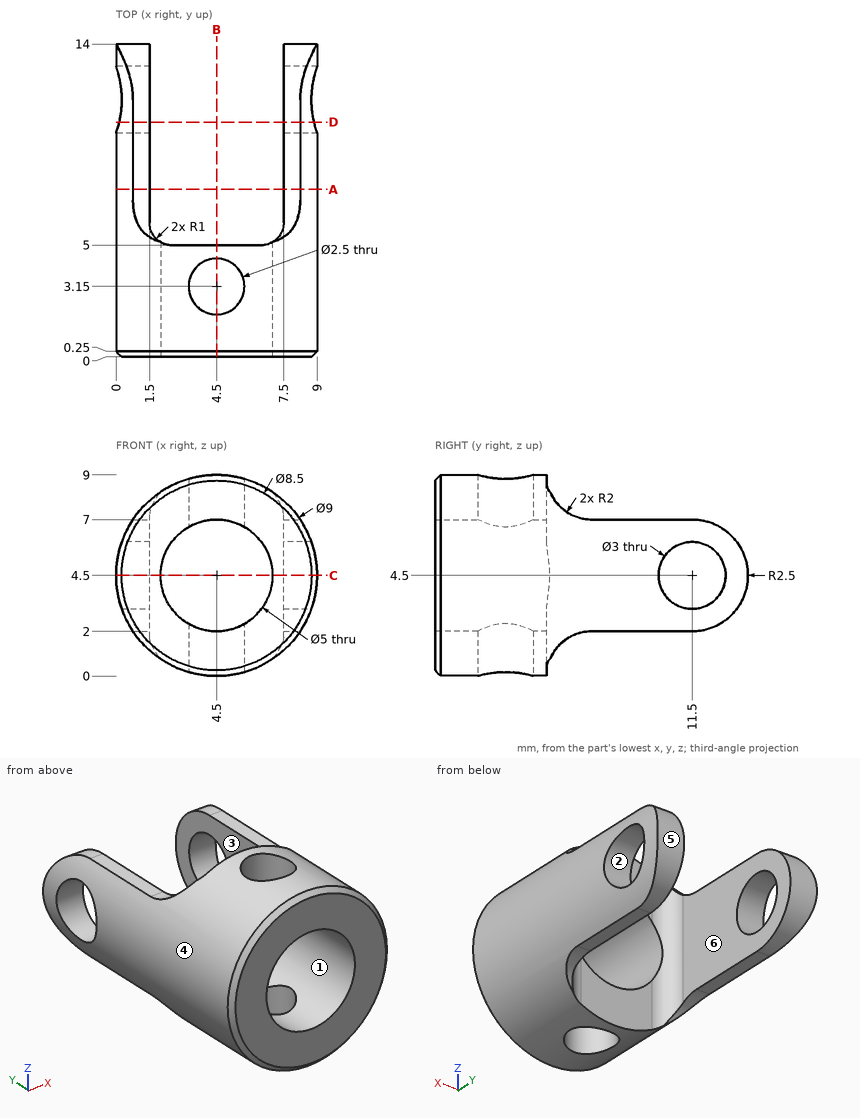
For this review, use the dimensioned drawing (mm, ordinates from the lowest corner) and the shaded views. A direction names the side the tool comes from. Round coordinates to 2 decimals unless told otherwise and drop trailing zeros. Write each loop counter-clockwise with the first axis right and the second up, starting at its lowest first coordinate (ties: lowest second). Pieces come first, ordered by that corner, then holes. Notation, with made-up numbers: (-31, 88) -> (-3, 88) arc R12 ccw to (-3, 107) -> close; hole circle Ø10 at (-16, -26.5). An arc over 180 degrees is marked (long way). One line per item, written item: value. Start each with the question number.
Q1. Insertion check: P1, Ø5, axis at y = 9.5, z = 1, coming from the +X side; P2, Ø2, axis at x = 4.5, y = 3.15, coming from the +Z side (3 decimals); P3, Ø1.5, axis at x = 4, z = 1.5, coming from the +Y side; P4, Ø0.8, axis at x = 1, y = 9, coming from the +Z side. Each pin has a flat end and moves straight along its axis. Give the tip position at first contact, or say it passes through.
Q2. Add section B-B (x = 4.5). Give the boundary of the cut face in (y, z).
Q3. To check wall thickness, follow probe 1 along X at (y, z) = (2.8, 4.5); probe 2 along Y at (x, z) = (0.85, 4.5); probe 3 along X at (y, z) = (1.5, 6.5). State the ranges of each line that lie inside material, in increasing order.
Q4. Tool access review of the marked faces 5 and 6: name each direction out of +Z, -Z, +X, -X, +Y, -Y from which nothing blocks a thin tool from reaching the whole face with its end or side.
Q5. Add section A-A (y = 7.5). Give the boundary of the cut face in (x, z).
Q6. The part is to be moulded in two halves that separate along Z. For the marked faces 1, 2, 3 and 4, say which applies: pulls with the +Z half, pulls with the -Z half, needs draft (parallel to the pull), parting line crosses it, or undercut.
Q7. Add section D-D (y = 10.5). Give the boundary of the cut face in (x, z).
Q8. Add section C-C (z = 4.5). Give the boundary of the cut face in (x, y), then the cut area to 3 significant figures.
Response:
1. P1: stops at x = 8.89
1. P2: passes through
1. P3: stops at y = 5
1. P4: stops at z = 7
2. outline: (0, 0.25) -> (0.25, 0) -> (1.9, 0) -> (1.9, 2) -> (0, 2) -> close; (0, 7) -> (1.9, 7) -> (1.9, 9) -> (0.25, 9) -> (0, 8.75) -> close; (4.4, 0) -> (5, 0) -> (5, 2) -> (4.4, 2) -> close; (4.4, 7) -> (5, 7) -> (5, 9) -> (4.4, 9) -> close
3. probe 1: x = 0 to 2, 7 to 9
3. probe 2: y = 0 to 10, 13 to 14
3. probe 3: x = 0.47 to 3, 6 to 8.53
4. face 5: +X, -X, +Y
4. face 6: +Z, -Z, +Y
5. outline: (0.76, 2) -> (1.5, 2) -> (1.5, 7) -> (0.76, 7) arc R4.5 ccw to start; (7.5, 2) -> (8.24, 2) arc R4.5 ccw to (8.24, 7) -> (7.5, 7) -> close
6. face 1: undercut
6. face 2: undercut
6. face 3: needs draft
6. face 4: parting line crosses it
7. outline: (0.14, 3.38) arc R4.5 ccw to (0.76, 2) -> (1.5, 2) -> (1.5, 3.38) -> close; (0.14, 5.62) -> (1.5, 5.62) -> (1.5, 7) -> (0.76, 7) arc R4.5 ccw to start; (7.5, 2) -> (8.24, 2) arc R4.5 ccw to (8.86, 3.38) -> (7.5, 3.38) -> close; (7.5, 5.62) -> (8.86, 5.62) arc R4.5 ccw to (8.24, 7) -> (7.5, 7) -> close
8. outline: (0, 0.25) -> (0.25, 0) -> (2, 0) -> (2, 5.13) arc R1 cw to (1.5, 6) -> (1.5, 10) -> (0, 10) -> close; (0, 13) -> (1.5, 13) -> (1.5, 14) -> (0, 14) -> close; (7, 0) -> (8.75, 0) -> (9, 0.25) -> (9, 10) -> (7.5, 10) -> (7.5, 6) arc R1 cw to (7, 5.13) -> close; (7.5, 13) -> (9, 13) -> (9, 14) -> (7.5, 14) -> close
8. area: 38.3 mm^2
